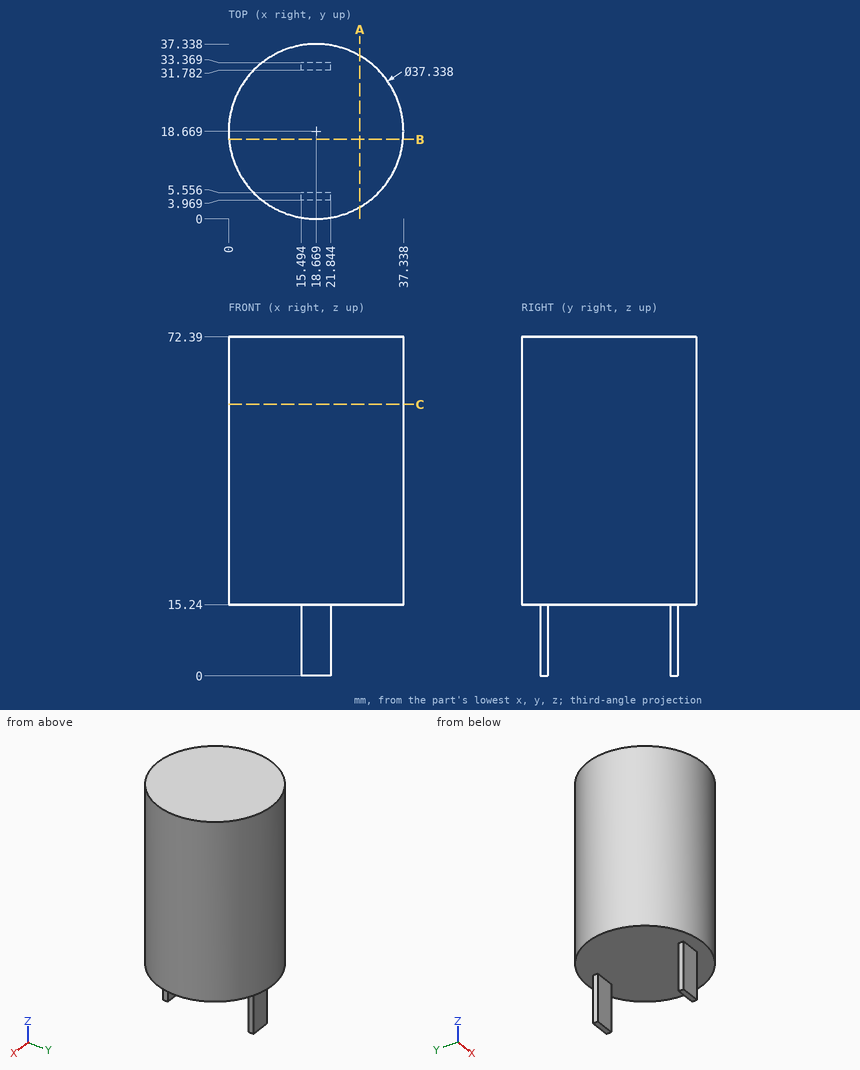
Geometry: see drawing. Coordinates: mm, zero at the bounding-box minimum. Round coordinates to 2 decimals unless told otherwise and drop trailing zeros. Order: outer loops, then holes, each group sorted by start corner. A loop starts at its lowest first (then second) coordinate and runs counter-clockwise, first axis right, second up. Notation, with made-up numbers: (88.5, -34) -> (106.5, -34) arc R18 ccw to (106.5, -10) -> close; hole circle Ø6 at (14.5, 62). An arc over 180 degrees is marked (long way). Answer as CSV lines item,"result".
Item 1: Section C-C, the plane z = 58. Return loops of the section in (x, y), plus the area to 4 significant figures.
A:
outline,"circle Ø37.34 at (18.67, 18.67)"
area,"1,095 mm²"
Item 2: Line query: L1, parallel to Z at x = 23, y = 30; L2, parallel to X at y = 18, z = 37.5; L3, parallel to Y at x = 33.5, z = 49.5. Output: solid intervals per line, ascending.
A:
L1,"15.24 to 72.39"
L2,"0.01 to 37.33"
L3,"7.33 to 30.01"
Item 3: Section B-B, the plane y = 17. Return loops of the section in (x, z) (1 decimal).
A:
outline,"(0.1, 15.2) -> (37.3, 15.2) -> (37.3, 72.4) -> (0.1, 72.4) -> close"
Item 4: Section A-A, the plane x = 28. Return loops of the section in (y, z), plus the area to 3 significant figures.
A:
outline,"(2.5, 15.24) -> (34.84, 15.24) -> (34.84, 72.39) -> (2.5, 72.39) -> close"
area,"1,850 mm²"
Item 5: Pin query (flat end, axial travel): pin 1 Ø1 at (y, z) = (17.5, 26.5) entering from +X; pin 2 Ø1.7 at (y, z) = (32.5, 9.5) entering from -X; pin 3 Ø1 at (x, z) = (4, 55) entering from +Y (1 decimal). Return the tip coordinate at first contact, or that it passes through.
A:
pin 1,"x = 37.33"
pin 2,"x = 15.49"
pin 3,"y = 30.8"
